Could you check a few things on this drawing? It's one solid part, dimensions in mm from its lowest x, y, z. Give positions to 0.01 mm unless a question says otherwise; leave off trailing zeros. Order: outer loops, then holes, each group sorted by start corner. A loop starts at its lowest first (then second) coordinate and runs counter-clockwise, first axis right, second up. Notation, with made-up numbers: M 21,45.5 L 48,45.5 A11 cw 48,58.5 Z; hole C -23,63.5 d4. An arc over 180 degrees is marked long. Use CSV: the item, a comma, the result in double quotes. Start each with the question number.
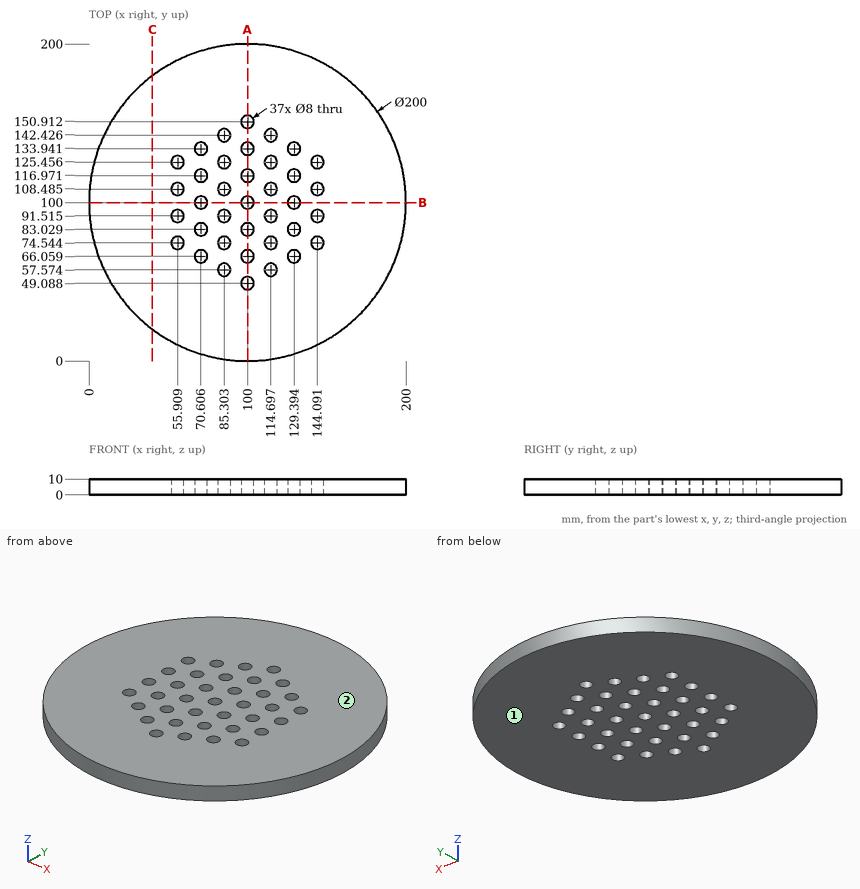
Q1. Imagine slicing it at A-A, the plane x = 100. Count the separate pieces of the cut face and the enclosed holes in it, then the cut area to 3 significant figures.
Q2. I need wall thicknesses on line 1 (X direction, y = 90, z = 5) (1 decimal); line 2 (X direction, y = 59, z = 2.25) (1 decimal); line 3 (X direction, y = 106, z = 2.5) (1 decimal). Which ranges of each line are inside material? Lowest first, please. Write a range as [from, to].
Q3. We'd pull the mould along Z, two halves only. Please class the marked faces 1 and 2: pulls with the +Z half, pulls with the -Z half, needs draft (parallel to the pull), parting line crosses it, or undercut.
Q4. For P1, Ø7, axis at x = 100, y = 66.06, coming from the +Z side; P2, Ø4, axis at y = 65, z = 8.5, coming from the -X side; P3, Ø5, axis at x = 61, z = 5, coming from the +Y side; P4, Ø1.5, axis at x = 169, z = 4, coming from the +Y side, each with a flat end and sliding along its axis, tell me the tip position at first contact or that it passes through.
Q5. Imagine slicing it at C-C, the plane x = 40. Please give me the cut outline in (y, z), then the cut area to 3 significant figures.
Q6. Imagine slicing it at B-B, the plane y = 100. Please give me the cut outline in (x, z).
Reply:
1,separate pieces,"8"
1,enclosed holes,"0"
1,area,"1,440 mm^2"
2,line 1,"x = [0.5, 52.2], [59.6, 81.6], [89, 111], [118.4, 140.4], [147.8, 199.5]"
2,line 2,"x = [8.8, 81.6], [89, 111], [118.4, 191.2]"
2,line 3,"x = [0.2, 52.8], [59, 82.2], [88.4, 111.6], [117.8, 141], [147.2, 199.8]"
3,face 1,"pulls with the -Z half"
3,face 2,"pulls with the +Z half"
4,P1,"passes through"
4,P2,"stops at x = 5.6"
4,P3,"stops at y = 193.1"
4,P4,"stops at y = 173.09"
5,outline,"M 20,0 L 180,0 L 180,10 L 20,10 Z"
5,area,"1,600 mm^2"
6,outline,"M 0,0 L 66.61,0 L 66.61,10 L 0,10 Z; M 74.61,0 L 96,0 L 96,10 L 74.61,10 Z; M 104,0 L 125.39,0 L 125.39,10 L 104,10 Z; M 133.39,0 L 200,0 L 200,10 L 133.39,10 Z"
